Can you work these out from the model? Positions are in its coordinate system, mm. Face numbers are marked on the shaded views. A direction names the side the tool comes from. Coordinates: 2 decimals unless noted, no trailing zeros. Loops run counter-clockwise (first coordinate to the right, second up) from the corner with the lowest first, then second, coordinate; pieces in that order, holes last. Notation, with made-up numbers: (-12, -37.5) - (12, -37.5) arc R26 ccw to (12, -16.5) - close; hole circle Ø11 at (19, 38). An arc over 180 degrees is marked (long way). Put each result on its own line as item: value. Start each with the question number.
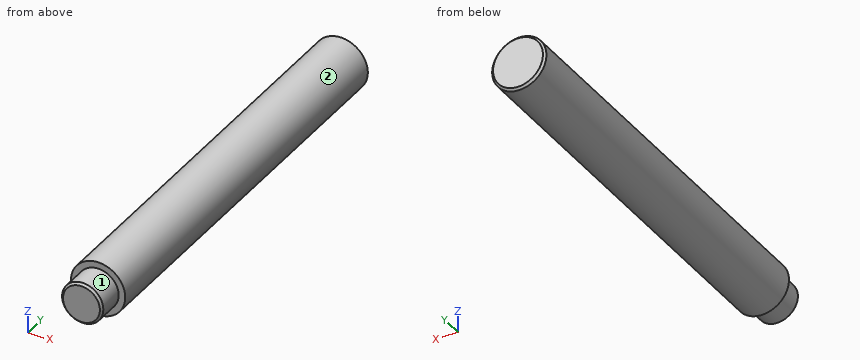
from build123d import *

# Parameters (mm, degrees)
F0_R     = 6.25
F1_DEPTH = 47.5
F2_R     = 4.75
F3_DEPTH = 6.5
F4_SIZE  = 0.5


with BuildPart() as f1:
    # F0 (on Front) → F1 (new body, symmetric)
    with BuildSketch(Plane.XZ):
        Circle(F0_R)
    extrude(amount=F1_DEPTH, both=True)

    # F2 (on face) → F3 (join)
    with BuildSketch(Plane.XZ.offset(47.5)):
        Circle(F2_R)
    extrude(amount=F3_DEPTH)

    # F4
    f4_edges = [f1.edges().sort_by_distance(p)[0] for p in [
        (-4.75, -54, 0),
        (-6.25, 47.5, 0),
    ]]
    chamfer(f4_edges, length=F4_SIZE)


solid = f1.part
Q1. Please list where these lines run through material, in increasing order: line 1 along Y through (x, z) = (4.5, -2.25); line 2 along Z through (x, y) = (0.25, 2.5) (3 decimals); line 3 along X through (y, z) = (-14, -4.5). Write a range as [from, to].
Q2. I want a section at B-B on x = 0. List the corners of the cut face in (y, z) for me.
Q3. On a 3-axis mill with a long thin cutter (end or side, diameter ignored), from which of +Z, -Z, +X, -X, +Y, -Y can I reach the whole of each face in a straight line? I mean the marked faces 1 and 2. Say none if no direction works.
Q4. Will these pins go through, and if not, where does the flat tip stop? pin 1 (3 mm diameter, centred on x = 2, y = -3.5, fed in from -Z); pin 2 (1 mm diameter, centred on y = 18.5, z = -2.5, fed in from +X); pin 3 (1.5 mm diameter, centred on x = 1.5, y = -37.5, fed in from +Z).
Q5. I want a section at C-C on y = 39.5. List the corners of the cut face in (x, z) for me.
Q6. I want a section at A-A on z = 0. List the corners of the cut face in (x, y) for me.
Calculated:
1. line 1: [-47.5, 47.5]
1. line 2: [-6.245, 6.245]
1. line 3: [-4.34, 4.34]
2. outline: (-54, -4.25) - (-53.5, -4.75) - (-47.5, -4.75) - (-47.5, -6.25) - (47, -6.25) - (47.5, -5.75) - (47.5, 5.75) - (47, 6.25) - (-47.5, 6.25) - (-47.5, 4.75) - (-53.5, 4.75) - (-54, 4.25) - close
3. face 1: -Y
3. face 2: +Y, -Y
4. pin 1: z = -6.23
4. pin 2: x = 5.92
4. pin 3: z = 6.2
5. outline: circle Ø12.5 at (0, 0)
6. outline: (-6.25, -47.5) - (-4.75, -47.5) - (-4.75, -53.5) - (-4.25, -54) - (4.25, -54) - (4.75, -53.5) - (4.75, -47.5) - (6.25, -47.5) - (6.25, 47) - (5.75, 47.5) - (-5.75, 47.5) - (-6.25, 47) - close
